CAD build for the part. Positions are in the model's coordinates, mm. Face numbers are marked on the shaded views. A direction names the side the tool comes from. Round coordinates to 2 decimals unless told otherwise and drop trailing zeros. Order: outer loops, then holes, each group sorted by start corner. A loop starts at its lowest first (then second) coordinate and runs counter-clockwise, first axis right, second up. Notation, with made-up numbers: (-22.5, 57) -> (32.5, 57) arc R21 cw to (32.5, 64) -> close; hole circle Ø8 at (25.5, -0.75). An arc over 180 degrees is marked (long way). Return JSON: item names as keys, results as strings. Group by question number.
Q1. Which spindle directions (+Z, -Z, +X, -X, +Y, -Y) get a long thin tool onto all of the face, cutting with end or side? Do the marked faces 1, 2 and 3. Say none if no direction does.
Q2. Mould opens along Z. For the marked faces 4, 5 and 6 say: +Z half, -Z half, draft (parallel to the pull), parting line (faces both ways), or undercut.
Q3. Cut at C-C (y = 8.5). Write the cut outline in (x, z) (1 decimal), then the cut area to 3 significant figures.
Q4. Cut at A-A (x = -7.5). Write the cut outline in (y, z) (3 decimals), then the cut area to 3 significant figures.
Q5. Cut at D-D (y = 26.5). Write the cut outline in (x, z) (1 decimal), then the cut area to 3 significant figures.
Q6. Probe line 1 along X through (y, z) = (20, -7); line 2 along Z through (x, y) = (12.7, 2) (3 decimals); line 3 along X through (y, z) = (21, -3.25). List the from-to ranges inside material, lowest first.
Q7. Flat gauge pins, fed straight in: pin 1 (4 mm diameter, centred on x = 0, z = -4.76, fed in from -Y); pin 2 (7 mm diameter, centred on x = 22.5, y = 20, fed in from +Z); pin 3 (7 mm diameter, centred on x = -22.5, y = 20, fed in from -Z) (3 decimals); pin 4 (2 mm diameter, centred on x = -7.5, z = -4.76, fed in from +Y). Where does each tip first touch, or does it go through?
Q8. Cut at B-B (z = -1.25). Write the cut outline in (x, y).
from build123d import *

# Parameters (mm, degrees)
F1_DEPTH = 9.525
F2_D     = 8.5
F2_DEPTH = 8
F2_TIP   = 2.5536576309
F4_D     = 5.1054
F4_DEPTH = 7.54
F4_TIP   = 1.5338169022
F6_D     = 3.4544
F6_DEPTH = 6.5875
F6_TIP   = 1.0378064612


with BuildPart() as f1:
    # F0 (on Top) → F1 (new body)
    with BuildSketch(Plane.XY):
        Polygon((-30, 0), (0, 0), (30, 0), (30, 30), (0, 30), (-30, 30), align=None)
    extrude(amount=-F1_DEPTH)

    # F2
    with Locations(Plane.XY):
        with Locations((-22.5, 20), (-7.5, 20), (7.5, 20), (22.5, 20)):
            Hole(F2_D / 2, depth=F2_DEPTH)
            with Locations((0, 0, -(F2_DEPTH + F2_TIP / 2))):  # 118° drill point
                Cone(0, F2_D / 2, F2_TIP, mode=Mode.SUBTRACT)

    # F4
    with Locations(Plane.XZ):
        with Locations((-25.4, -4.7625), (-12.7, -4.7625), (0, -4.7625), (12.7, -4.7625), (25.4, -4.7625)):
            Hole(F4_D / 2, depth=F4_DEPTH)
            with Locations((0, 0, -(F4_DEPTH + F4_TIP / 2))):  # 118° drill point
                Cone(0, F4_D / 2, F4_TIP, mode=Mode.SUBTRACT)

    # F6
    with Locations(Plane(origin=(0, 30, 0), x_dir=(-1, 0, 0), z_dir=(0, 1, 0))):
        with Locations((-22.5, -4.7625), (-7.5, -4.7625), (7.5, -4.7625), (22.5, -4.7625)):
            Hole(F6_D / 2, depth=F6_DEPTH)
            with Locations((0, 0, -(F6_DEPTH + F6_TIP / 2))):  # 118° drill point
                Cone(0, F6_D / 2, F6_TIP, mode=Mode.SUBTRACT)


solid = f1.part
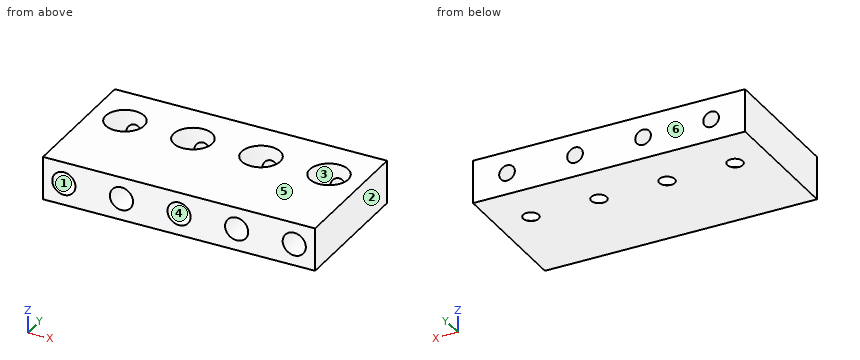
Solution:
{
 "1": {"face 1": "-Y", "face 2": "+Z, -Z, +X, +Y, -Y", "face 3": "+Z"},
 "2": {"face 4": "undercut", "face 5": "+Z half", "face 6": "draft"},
 "3": {"outline": "(-30, -9.5) -> (30, -9.5) -> (30, 0) -> (-30, 0) -> close; hole circle Ø1.9 at (-25.4, -4.8); hole circle Ø1.9 at (-12.7, -4.8); hole circle Ø1.9 at (0, -4.8); hole circle Ø1.9 at (12.7, -4.8); hole circle Ø1.9 at (25.4, -4.8)", "area": "557 mm²"},
 "4": {"outline": "(0, -9.525) -> (18.288, -9.525) -> (15.75, -8) -> (15.75, 0) -> (0, 0) -> close; (21.712, -9.525) -> (30, -9.525) -> (30, -6.49) -> (24.25, -6.49) -> (24.25, -8) -> close; (24.25, -3.035) -> (30, -3.035) -> (30, 0) -> (24.25, 0) -> close", "area": "189 mm²"},
 "5": {"outline": "(-30, -9.5) -> (30, -9.5) -> (30, 0) -> (-30, 0) -> close; hole circle Ø3.5 at (-22.5, -4.8); hole circle Ø3.5 at (-7.5, -4.8); hole circle Ø3.5 at (7.5, -4.8); hole circle Ø3.5 at (22.5, -4.8)", "area": "534 mm²"},
 "6": {"line 1": "x = -30 to -26.75, -18.25 to -11.75, -3.25 to 3.25, 11.75 to 18.25, 26.75 to 30", "line 2": "z = -9.525 to -7.315, -2.21 to 0", "line 3": "x = -30 to -26.63, -18.37 to -11.63, -3.37 to 3.37, 11.63 to 18.37, 26.63 to 30"},
 "7": {"pin 1": "stops at y = 7.87", "pin 2": "stops at z = -8.45", "pin 3": "stops at z = -9.525", "pin 4": "stops at y = 15.87"},
 "8": {"outline": "(-30, 0) -> (30, 0) -> (30, 30) -> (-30, 30) -> close; hole circle Ø8.5 at (-22.5, 20); hole circle Ø8.5 at (-7.5, 20); hole circle Ø8.5 at (7.5, 20); hole circle Ø8.5 at (22.5, 20)"}
}
